from build123d import *

# Parameters (mm, degrees)
SKETCH1_R           = 15.125
SKETCH1_R_2         = 10
BOSS_EXTRUDE1_DEPTH = 7.5
SKETCH2_R           = 5.25
FILLET1_R           = 1


with BuildPart() as part:
    # Sketch1 → Boss-Extrude1 (new, symmetric)
    with BuildSketch(Plane(origin=(0, 0, 0), x_dir=(0, 0, -1), z_dir=(1, 0, 0))):
        Circle(SKETCH1_R)
        Circle(SKETCH1_R_2, mode=Mode.SUBTRACT)
    extrude(amount=BOSS_EXTRUDE1_DEPTH, both=True)

    # Sketch2 → Cut-Revolve1 (revolve, cut)
    with BuildSketch(Plane.XY, mode=Mode.PRIVATE) as cut_revolve1_sk:
        with Locations((0, 18.5)):
            Circle(SKETCH2_R)
    revolve(cut_revolve1_sk.sketch.rotate(Axis((0, 0, 0), (1, 0, 0)), 90), axis=Axis((0, 0, 0), (1, 0, 0)), mode=Mode.SUBTRACT)

    # Fillet1
    fillet1_edges = [part.edges().sort_by_distance(p)[0] for p in [
        (-7.5, 0, 10),
        (7.5, 0, 10),
    ]]
    fillet(fillet1_edges, radius=FILLET1_R)


solid = part.part
The listing builds one solid part. Answer for the finished solid, in the listing's coordinates (mm). Coordinates: 2 decimals unless noted, no trailing zeros. Loops run counter-clockwise (first coordinate to the right, second up) from the corner with the lowest first, then second, coordinate; pieces in that order, holes last.
1) Find section A-A on y = 0. Write down the section's boundary in (x, z) (3 decimals), then the cut area to 3 significant figures.
2) Flat-ended cylindrical pins translate along their axes: pin 1 Ø6 at (x, y) = (6, 10) entering from -Z; pin 2 Ø4 at (x, y) = (-1, 5.5) entering from +Z; pin 3 Ø3 at (x, y) = (-3.5, 7.5) entering from +Z; pin 4 Ø10 at (y, z) = (-4.5, -0.5) entering from +X (3 decimals). Find the tip coordinate at first contact, or state that the pin passes through.
3) Find section C-C on x = -5. Write down the section's boundary in (y, z) (3 decimals).
4) Find section D-D on x = 2.75. Write down the section's boundary in (y, z), then the cut area to 3 significant figures.
5) Determine the mould class of faces 1 (the face through (7.5, -11.13, -1.05)), 2 (the face through (-0.09, -9.76, 2.17)), 3 (the face through (5.785, -14.765, 3.279)) for opening direction Z: pulls with the +Z half, pulls with the -Z half, needs draft (parallel to the pull), parting line crosses it, or undercut.
6) Find the intervals of material crossed by L1, parallel to Y at x = 4.25, z = 0 (3 decimals); L2, parallel to Z at x = 4, y = -7; L3, parallel to Y at x = -2.75, z = 7, in increasing order.
Values:
1. outline: (-7.5, -15.125) - (-4.021, -15.125) arc R5.25 cw to (4.021, -15.125) - (7.5, -15.125) - (7.5, -11) arc R1 ccw to (6.5, -10) - (-6.5, -10) arc R1 ccw to (-7.5, -11) - close; (-7.5, 11) arc R1 ccw to (-6.5, 10) - (6.5, 10) arc R1 ccw to (7.5, 11) - (7.5, 15.125) - (4.021, 15.125) arc R5.25 cw to (-4.021, 15.125) - (-7.5, 15.125) - close
1. area: 132 mm2
2. pin 1: stops at z = -13.41
2. pin 2: stops at z = 13.28
2. pin 3: stops at z = 13.84
2. pin 4: passes through
3. outline: circle Ø30.25 at (0, 0); hole circle Ø20 at (0, 0)
4. outline: circle Ø28.06 at (0, 0); hole circle Ø20 at (0, 0)
4. area: 304 mm2
5. face 1: needs draft
5. face 2: undercut
5. face 3: parting line crosses it
6. L1: y = -15.125 to -10, 10 to 15.125
6. L2: z = -13.38 to -7.14, 7.14 to 13.38
6. L3: y = -12.16 to -7.14, 7.14 to 12.16
